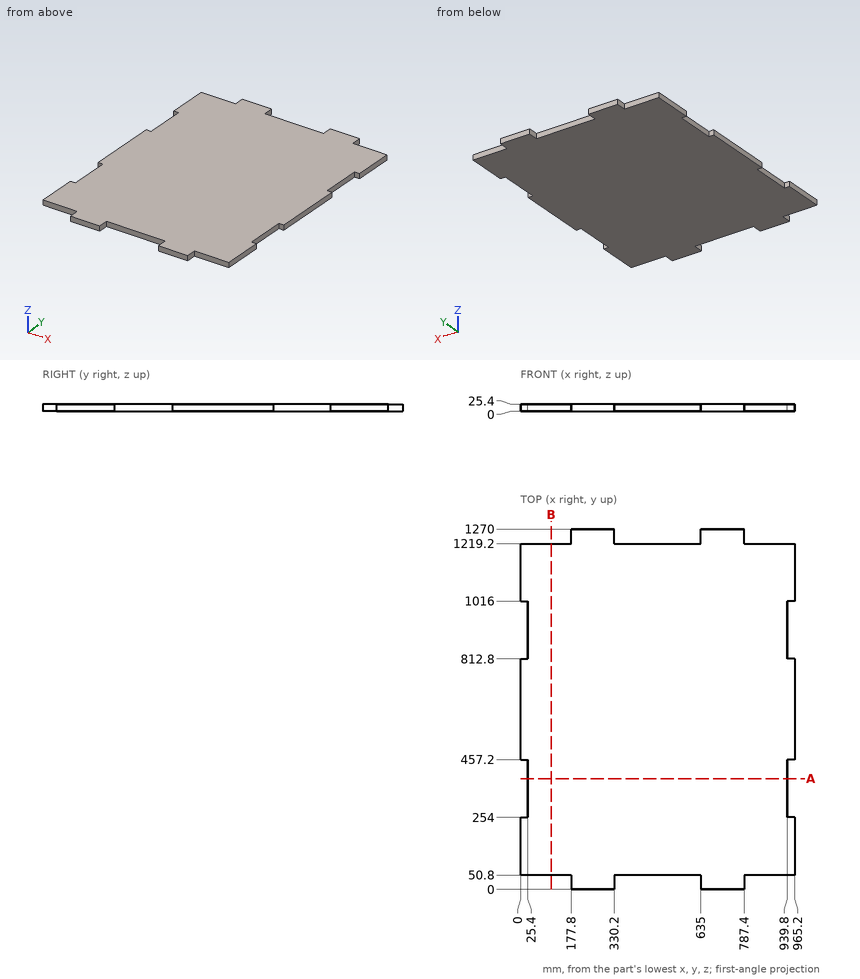
Source: three-view drawing plus pictorial views. Frame: mm from the lowest corner of the part. Round coordinates to 2 decimals unless told otherwise and drop trailing zeros. Loops run counter-clockwise (first coordinate to the right, second up) from the corner with the lowest first, then second, coordinate; pieces in that order, holes last.
Q1. Section A-A, the plane y = 390.5. Return loops of the section in (x, z), plus the area to 3 significant figures.
Q2. First-contact query: P1, Ø7.5, axis at y = 37, z = 15.5, coming from the +X side; P2, Ø6, axis at x = 328.5, z = 22, coming from the -Y side; P3, Ø7.5, axis at y = 937, z = 15.5, coming from the +X side; P4, Ø12.5, axis at x = 955, z = 6.5, coming from the +Y side. Flat tips, straight axial feed; report the tip coordinate or a pass-through.
Q3. Ray query, line 1 (X direction, y = 854, z = 8.25); line 2 (Y direction, x = 831.5, z = 21). Return the intervals inside material, ascending.
Q4. Section B-B, the plane x = 107. Return loops of the section in (y, z), plus the area to 3 significant figures.
Solutions:
1. outline: (25.4, 0) - (939.8, 0) - (939.8, 25.4) - (25.4, 25.4) - close
1. area: 23,200 mm2
2. P1: stops at x = 787.4
2. P2: stops at y = 0
2. P3: stops at x = 939.8
2. P4: stops at y = 1219.2
3. line 1: x = 25.4 to 939.8
3. line 2: y = 50.8 to 1219.2
4. outline: (50.8, 0) - (1219.2, 0) - (1219.2, 25.4) - (50.8, 25.4) - close
4. area: 29,700 mm2
